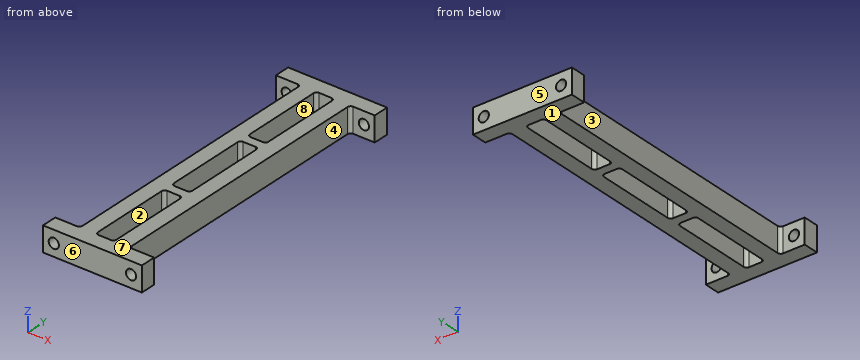
```python
from build123d import *

# Parameters (mm, degrees)
EXTRUDE_1_DEPTH     = 8
FILLET_1_R          = 1
SKETCH_3_W          = 6
SKETCH_3_H          = 90
CUT_EXTRUDE_2_DEPTH = 10
FILLET_2_R          = 1
HOLE_WIZARD_M4_1_D  = 3.3
SKETCH_6_W          = 6
SKETCH_6_H          = 3
EXTRUDE_2_DEPTH     = 8
FILLET_3_R          = 1


with BuildPart() as part:
    # 草图1 → 凸台-拉伸1 (new body)
    with BuildSketch(Plane.XY):
        Polygon((8, 45), (8, -45), (16, -45), (16, -50), (-16, -50), (-16, -45), (-8, -45), (-8, 45), (-16, 45), (-16, 50), (16, 50), (16, 45), align=None)
    extrude(amount=EXTRUDE_1_DEPTH)

    # 圆角1
    fillet_1_edges = [part.edges().sort_by_distance(p)[0] for p in [
        (8, -45, 4),
        (-8, -45, 4),
        (-8, 45, 4),
        (8, 45, 4),
    ]]
    fillet(fillet_1_edges, radius=FILLET_1_R)

    # 草图3 → 切除-拉伸2 (cut)
    with BuildSketch(Plane.XY.offset(8)):
        Rectangle(SKETCH_3_W, SKETCH_3_H)
    extrude(amount=-CUT_EXTRUDE_2_DEPTH, mode=Mode.SUBTRACT)

    # 圆角2
    fillet_2_edges = [part.edges().sort_by_distance(p)[0] for p in [
        (3, 45, 4),
        (3, -45, 4),
        (-3, -45, 4),
        (-3, 45, 4),
    ]]
    fillet(fillet_2_edges, radius=FILLET_2_R)

    # M4 螺纹孔的螺纹孔钻头1 (through all)
    with Locations(Plane(origin=(0, -50, 0), x_dir=(-1, 0, 0), z_dir=(0, -1, 0))):
        with Locations((-12.5, -4), (12.5, -4)):
            Hole(HOLE_WIZARD_M4_1_D / 2)

    # 草图6 → 凸台-拉伸2 (add)
    with BuildSketch(Plane(origin=(0, 0, 0), x_dir=(-1, 0, 0), z_dir=(0, 0, -1))):
        with Locations((0, 15.5)):
            Rectangle(SKETCH_6_W, SKETCH_6_H)
        with Locations((0, -15.5)):
            Rectangle(SKETCH_6_W, SKETCH_6_H)
    extrude(amount=-EXTRUDE_2_DEPTH)

    # 圆角3
    fillet_3_edges = [part.edges().sort_by_distance(p)[0] for p in [
        (3, 17, 4),
        (3, 14, 4),
        (-3, 14, 4),
        (-3, 17, 4),
        (3, -14, 4),
        (3, -17, 4),
        (-3, -17, 4),
        (-3, -14, 4),
    ]]
    fillet(fillet_3_edges, radius=FILLET_3_R)


solid = part.part
```
Verification items for the finished model (mm, model axes). Face numbers are marked on the shaded views. A direction names the side the tool comes from. Give positions to 0.01 mm unless a question says otherwise; leave off trailing zeros. Order: outer loops, then holes, each group sorted by start corner. A loop starts at its lowest first (then second) coordinate and runs counter-clockwise, first axis right, second up. Notation, with made-up numbers: (-25.5, -25.5) -> (13.5, -25.5) arc R11 ccw to (13.5, -8.5) -> close; hole circle Ø1 at (48, 45). An arc over 180 degrees is marked (long way). Use a Markdown table: item, result.
1) Tool access check on the marked faces 1, 2, 3 and 4. Record the directions out of +Z, -Z, +X, -X, +Y, -Y that give a thin tool (end or side, any length) a straight path to the whole face; none if there is none.
Results:
| item | result |
|---|---|
| face 1 | -Z, +X, -X, +Y, -Y |
| face 2 | +Z, -Z |
| face 3 | +Z, -Z, -X |
| face 4 | +Z, -Z, +X |
2) Section check C-C, the plane z = 4. Give the number of separate pieces and of enclosed holes in the cut face, then the cut area to 3 significant figures.
Results:
| item | result |
|---|---|
| separate pieces | 5 |
| enclosed holes | 3 |
| area | 1,190 mm² |
3) Section check A-A, the plane x = 12.5. Record the boundary of the cut face in (y, z), then the cut area to 3 significant figures.
Results:
| item | result |
|---|---|
| outline | (-50, 0) -> (-45, 0) -> (-45, 2.35) -> (-50, 2.35) -> close; (-50, 5.65) -> (-45, 5.65) -> (-45, 8) -> (-50, 8) -> close; (45, 0) -> (50, 0) -> (50, 2.35) -> (45, 2.35) -> close; (45, 5.65) -> (50, 5.65) -> (50, 8) -> (45, 8) -> close |
| area | 47.0 mm² |
4) Depth check by flat-ended pin: pin 1 Ø4 at (x, y) = (-11, -29.5) entering from +Z; pin 2 Ø4 at (y, z) = (-19, 7) entering from -X; pin 3 Ø1 at (y, z) = (-28, 4.5) entering from +X. Enter the tip coordinate at first touch or a pass-through.
Results:
| item | result |
|---|---|
| pin 1 | through |
| pin 2 | x = -8 |
| pin 3 | x = 8 |
5) Material ranges on probe 1 along X at (y, z) = (48.55, 4); probe 2 along Y at (x, z) = (0.5, 5.25); probe 3 along X at (y, z) = (-23.5, 0.75), recorded low to high.
Results:
| item | result |
|---|---|
| probe 1 | -16 to -14.15, -10.85 to 10.85, 14.15 to 16 |
| probe 2 | -50 to -45, -17 to -14, 14 to 17, 45 to 50 |
| probe 3 | -8 to -3, 3 to 8 |
6) Mould release check, pull along Y, two halves, no side actions. Record for the marked faces 5, 6, 7 and 8: pulls with the +Y half, pulls with the -Y half, needs draft (parallel to the pull), parting line crosses it, or undercut.
Results:
| item | result |
|---|---|
| face 5 | pulls with the +Y half |
| face 6 | pulls with the -Y half |
| face 7 | needs draft |
| face 8 | undercut |
7) Section check B-B, the plane y = -20. Record the boundary of the cut face in (x, z), then the cut area to 3 significant figures.
Results:
| item | result |
|---|---|
| outline | (-8, 0) -> (-3, 0) -> (-3, 8) -> (-8, 8) -> close; (3, 0) -> (8, 0) -> (8, 8) -> (3, 8) -> close |
| area | 80.0 mm² |
8) Section check D-D, the plane x = 1. Record the boundary of the cut face in (y, z).
Results:
| item | result |
|---|---|
| outline | (-50, 0) -> (-45, 0) -> (-45, 8) -> (-50, 8) -> close; (-17, 0) -> (-14, 0) -> (-14, 8) -> (-17, 8) -> close; (14, 0) -> (17, 0) -> (17, 8) -> (14, 8) -> close; (45, 0) -> (50, 0) -> (50, 8) -> (45, 8) -> close |
